from build123d import *

# Parameters (mm, degrees)
SKETCH1_W                  = 5
SKETCH1_H                  = 110
BOSS_EXTRUDE1_DEPTH        = 120
BOSS_EXTRUDE1_DEPTH_BACK   = 110
BOSS_EXTRUDE1_2_DEPTH      = 120
BOSS_EXTRUDE1_2_DEPTH_BACK = 110
SKETCH2_W                  = 5
SKETCH2_H                  = 37
BOSS_EXTRUDE2_DEPTH        = 50
SKETCH3_W                  = 220
SKETCH3_H                  = 5
BOSS_EXTRUDE3_DEPTH        = 50
SKETCH4_W                  = 230
SKETCH4_H                  = 73
BOSS_EXTRUDE6_DEPTH        = 5
FILLET3_R                  = 15
CUT_EXTRUDE3_DEPTH         = 231
SKETCH5_W                  = 348
SKETCH5_H                  = 227
SKETCH5_W_2                = 328
SKETCH5_H_2                = 207
BOSS_EXTRUDE7_DEPTH        = 5
BOSS_EXTRUDE8_DEPTH        = 59
FILLET5_R                  = 15
BOSS_EXTRUDE9_DEPTH        = 5
BOSS_EXTRUDE10_DEPTH       = 5
FILLET6_R                  = 3
CUT_EXTRUDE4_DEPTH         = 60
CUT_EXTRUDE4_DEPTH_BACK    = 290
SKETCH15_R                 = 1.2
CUT_EXTRUDE5_DEPTH         = 16
SKETCH18_R                 = 3
CUT_EXTRUDE6_DEPTH         = 9


with BuildPart() as part:
    # Sketch1 → Boss-Extrude1 (new body, two sides)
    with BuildSketch(Plane(origin=(0, 0, 0), x_dir=(0, 0, -1), z_dir=(1, 0, 0))) as boss_extrude1_sk:
        with Locations((-112.5, 55)):
            Rectangle(SKETCH1_W, SKETCH1_H)
    extrude(amount=BOSS_EXTRUDE1_DEPTH)
    extrude(boss_extrude1_sk.sketch, amount=-BOSS_EXTRUDE1_DEPTH_BACK)



with BuildPart() as body_2:
    # Sketch1 → Boss-Extrude1 2 (new body, two sides)
    with BuildSketch(Plane(origin=(0, 0, 0), x_dir=(0, 0, -1), z_dir=(1, 0, 0))) as boss_extrude1_2_sk:
        with Locations((112.5, 55)):
            Rectangle(SKETCH1_W, SKETCH1_H)
    extrude(amount=BOSS_EXTRUDE1_2_DEPTH)
    extrude(boss_extrude1_2_sk.sketch, amount=-BOSS_EXTRUDE1_2_DEPTH_BACK)


with BuildPart() as part_1:
    add(part.part)

    add(body_2.part)  # Boss-Extrude2 merges body 2
    # Sketch2 → Boss-Extrude2 (add)
    with BuildSketch(Plane.ZY.offset(110)):
        with Locations((-112.5, 18.5)):
            Rectangle(SKETCH2_W, SKETCH2_H)
        with Locations((112.5, 18.5)):
            Rectangle(SKETCH2_W, SKETCH2_H)
    extrude(amount=BOSS_EXTRUDE2_DEPTH)

    # Sketch3 → Boss-Extrude3 (add)
    with BuildSketch(Plane.ZY.offset(160)):
        with Locations((0, 34.5)):
            Rectangle(SKETCH3_W, SKETCH3_H)
    extrude(amount=-BOSS_EXTRUDE3_DEPTH)

    # Sketch4 → Boss-Extrude6 (add)
    with BuildSketch(Plane.ZY.offset(110)):
        with Locations((0, 73.5)):
            Rectangle(SKETCH4_W, SKETCH4_H)
    extrude(amount=BOSS_EXTRUDE6_DEPTH)

    # Fillet3
    fillet3_edges = [part_1.edges().sort_by_distance(p)[0] for p in [
        (-115, 37, 0),
    ]]
    fillet(fillet3_edges, radius=FILLET3_R)

    # Sketch9 → Cut-Extrude3 (cut, through all)
    with BuildSketch(Plane.XY.offset(115)):
        Polygon((120, 110), (116.464466094, 106.464466094), (120, 102.928932188), align=None)
    extrude(amount=-CUT_EXTRUDE3_DEPTH, mode=Mode.SUBTRACT)

    # Sketch10 → Boss-Extrude8 (add)
    with BuildSketch(Plane.XY.offset(115)):
        Polygon((120, 110), (111.464466094, 110), (111.464466094, 0), (120, 0), (120, 102.928932188), (116.464466094, 106.464466094), align=None)
    boss_extrude8 = extrude(amount=BOSS_EXTRUDE8_DEPTH)

    # Mirror3: Boss-Extrude8 across plane
    add(boss_extrude8.mirror(Plane.XY))

    # Fillet5
    fillet5_edges = [part_1.edges().sort_by_distance(p)[0] for p in [
        (111.464466094, 55, 115),
        (111.464466094, 55, -115),
    ]]
    fillet(fillet5_edges, radius=FILLET5_R)

    # Fillet6
    fillet6_edges = [part_1.edges().sort_by_distance(p)[0] for p in [
        (111.464466094, 55, 174),
        (111.464466094, 55, -174),
    ]]
    fillet(fillet6_edges, radius=FILLET6_R)


with BuildPart() as body_2_2:
    # Sketch5 → Boss-Extrude7 (new body)
    with BuildSketch(Plane(origin=(115, 115, 0), x_dir=(0, 0, 1), z_dir=(-0.707106781, -0.707106781, 0))):
        with Locations((0, -120.571067812)):
            Rectangle(SKETCH5_W, SKETCH5_H)
        with Locations((0, -120.571067812)):
            Rectangle(SKETCH5_W_2, SKETCH5_H_2, mode=Mode.SUBTRACT)
    extrude(amount=BOSS_EXTRUDE7_DEPTH)


with BuildPart() as body_3:
    # Sketch12 → Boss-Extrude9 (new body)
    with BuildSketch(Plane.XY.offset(174)):
        Polygon((120, 0), (222.928932188, 0), (120, 102.928932188), align=None)
    extrude(amount=-BOSS_EXTRUDE9_DEPTH)


with BuildPart() as body_4:
    # Sketch13 → Boss-Extrude10 (new body)
    with BuildSketch(Plane(origin=(0, 0, -174), x_dir=(-1, 0, 0), z_dir=(0, 0, -1))):
        Polygon((-120, 102.928932188), (-120, 0), (-222.928932188, 0), align=None)
    extrude(amount=-BOSS_EXTRUDE10_DEPTH)


with BuildPart() as cut_extrude4_tool:
    # Sketch14 → Cut-Extrude4 (new body, two sides)
    with BuildSketch(Plane.XY.offset(115)) as cut_extrude4_sk:
        Polygon((-130, 37), (-115, 37), (-115, 120.163626998), (321.994934014, 120.163626998), (321.994934014, -84.01084078), (-160, -84.01084078), (-160, 37), align=None)
    extrude(amount=CUT_EXTRUDE4_DEPTH)
    extrude(cut_extrude4_sk.sketch, amount=-CUT_EXTRUDE4_DEPTH_BACK)


with BuildPart() as part_2:
    add(part_1.part)

    # Cut-Extrude4: cut by cut_extrude4_tool
    add(cut_extrude4_tool.part, mode=Mode.SUBTRACT)

    # Sketch15 → Cut-Extrude5 (cut, through all)
    with BuildSketch(Plane.XZ.offset(-37)):
        with Locations((-121, -70)):
            Circle(SKETCH15_R)
        with Locations((-121, 70)):
            Circle(SKETCH15_R)
    extrude(amount=-CUT_EXTRUDE5_DEPTH, mode=Mode.SUBTRACT)

    # Sketch18 → Cut-Extrude6 (cut)
    with BuildSketch(Plane(origin=(0, 47, 0), x_dir=(-1, 0, 0), z_dir=(0, -1, 0))):
        with Locations((121, 70)):
            Circle(SKETCH18_R)
        with Locations((121, -70)):
            Circle(SKETCH18_R)
    extrude(amount=CUT_EXTRUDE6_DEPTH, mode=Mode.SUBTRACT)


with BuildPart() as body_2_2_1:
    add(body_2_2.part)

    # Cut-Extrude4: cut by cut_extrude4_tool
    add(cut_extrude4_tool.part, mode=Mode.SUBTRACT)


with BuildPart() as body_3_1:
    add(body_3.part)

    # Cut-Extrude4: cut by cut_extrude4_tool
    add(cut_extrude4_tool.part, mode=Mode.SUBTRACT)


with BuildPart() as body_4_1:
    add(body_4.part)

    # Cut-Extrude4: cut by cut_extrude4_tool
    add(cut_extrude4_tool.part, mode=Mode.SUBTRACT)


solid = part_2.part
Part model, mm, in its own coordinate system. A direction names the side the tool comes from. Coordinates: 2 decimals unless noted, no trailing zeros. Write each loop counter-clockwise with the first axis right and the second up, starting at its lowest first coordinate (ties: lowest second). Pieces come first, ordered by that corner, then holes. Notation, with made-up numbers: M 38.5,9.5 L 46.5,9.5 A28 cw 46.5,40.5 Z; hole C 56,67.5 d11. An arc over 180 degrees is marked long. Return JSON: item names as keys, results as strings.
1. Probe L1, parallel to Z at x = -121, y = 39.9; L2, parallel to X at y = 43, z = -86.5; L3, parallel to Y at x = -124.5, z = -58. List the from-to ranges inside material, lowest first.
Determined:
{"L1": "-115 to -73, -67 to 67, 73 to 115", "L2": "-118 to -115", "L3": "37 to 38.04"}
2. Saw through at B-B, the plane y = 49.5. Write the cut outline in (x, z).
Determined:
{"outline": "M -115.21,-115 L -115,-115 L -115,115 L -115.21,115 Z"}
3. Flat gauge pins, fed straight in: pin 1 Ø5 at (x, z) = (-122.5, -70) entering from +Y; pin 2 Ø8 at (y, z) = (43, 43.5) entering from -X; pin 3 Ø3 at (x, z) = (-121.5, 91.5) entering from +Y. Where does each tip first touch, or does it go through?
Determined:
{"pin 1": "y = 38.91", "pin 2": "x = -122.52", "pin 3": "y = 40.82"}
4. Pull direction X, two halves, no side cores. Call faces 3 (the face through (-122, 38, 71)), 4 (the face through (-119.28, 41.51, 1.61)), 5 (the face through (-115, 44, 2)), 6 (the face through (-122, 37, 2)): pulls with the +X half, pulls with the -X half, needs draft (parallel to the pull), parting line crosses it, or undercut.
Determined:
{"face 3": "undercut", "face 4": "pulls with the -X half", "face 5": "pulls with the +X half", "face 6": "needs draft"}
5. 3-axis set-ups, long thin cutter, end or side, ignore diameter. For faces 1 (the face through (-119, 40, 115)), 2 (the face through (-118, 40, -70)): which of +Z, -Z, +X, -X, +Y, -Y reach the whole face in a straight line?
Determined:
{"face 1": "+Z, +X, -X, +Y, -Y", "face 2": "+Y"}
6. Saw through at A-A, the plane z = -50. Write the cut outline in (x, y), then the cut area to 3 significant figures.
Determined:
{"outline": "M -130,37 L -115,37 L -115,52 A15 cw Z", "area": "48.3 mm²"}
